```python
from build123d import *

# Parameters (mm, degrees)
SKETCH_1_W             = 162
SKETCH_1_H             = 108
EXTRUDE_1_DEPTH        = 3
SKETCH_2_R             = 2
SKETCH_2_W             = 42
SKETCH_2_H             = 7.5
SKETCH_2_W_2           = 27
SKETCH_2_W_3           = 32
SKETCH_2_W_4           = 58
SKETCH_2_H_2           = 5.8
SKETCH_2_W_5           = 69
SKETCH_2_H_3           = 24
SKETCH_2_W_6           = 13
SKETCH_2_H_4           = 13
CUT_EXTRUDE_2448_DEPTH = 4
FILLET_1_R             = 1.5
SKETCH_3_R             = 1.25
CUT_EXTRUDE_3312_DEPTH = 4
SKETCH_4_R             = 2
CUT_EXTRUDE_4190_DEPTH = 4
FILLET_2_R             = 2


with BuildPart() as part:
    # Эскиз1 → Бобышка-Вытянуть1 (new body)
    with BuildSketch(Plane(origin=(0, 0, 0), x_dir=(1, 0, 0), z_dir=(0, 1, 0))):
        Rectangle(SKETCH_1_W, SKETCH_1_H)
    extrude(amount=EXTRUDE_1_DEPTH)

    # Эскиз2 → Cut-Extrude 2448 (cut, through all)
    with BuildSketch(Plane(origin=(0, 3, 0), x_dir=(1, 0, 0), z_dir=(0, 1, 0))):
        with Locations((-72.99950864, 44.00008818)):
            Circle(SKETCH_2_R)
        with Locations((73, 44)):
            Circle(SKETCH_2_R)
        with Locations((-73, -44)):
            Circle(SKETCH_2_R)
        with Locations((73, -44)):
            Circle(SKETCH_2_R)
        with Locations((-0.725, 38)):
            Rectangle(SKETCH_2_W, SKETCH_2_H)
        with Locations((-31.975, 23)):
            Rectangle(SKETCH_2_W_2, SKETCH_2_H)
        with Locations((31.475, 14)):
            Rectangle(SKETCH_2_W_3, SKETCH_2_H)
        with Locations((0.475, 0)):
            Rectangle(SKETCH_2_W_4, SKETCH_2_H_2)
        with Locations((3, -27)):
            Rectangle(SKETCH_2_W_5, SKETCH_2_H_3)
        with Locations((48.316, -7.9)):
            Rectangle(SKETCH_2_W_6, SKETCH_2_H_4)
    extrude(amount=-CUT_EXTRUDE_2448_DEPTH, mode=Mode.SUBTRACT)

    # Скругление1
    fillet_1_edges = [part.edges().sort_by_distance(p)[0] for p in [
        (-31.5, 1.5, 39),
        (-31.5, 1.5, 15),
        (37.5, 1.5, 15),
        (37.5, 1.5, 39),
    ]]
    fillet(fillet_1_edges, radius=FILLET_1_R)

    # Эскиз3 → Cut-Extrude 3312 (cut, through all)
    with BuildSketch(Plane(origin=(0, 3, 0), x_dir=(1, 0, 0), z_dir=(0, 1, 0))):
        with Locations((-57, 42)):
            Circle(SKETCH_3_R)
        with Locations((-57, -10)):
            Circle(SKETCH_3_R)
        with Locations((60, 42)):
            Circle(SKETCH_3_R)
        with Locations((60, -10)):
            Circle(SKETCH_3_R)
    extrude(amount=-CUT_EXTRUDE_3312_DEPTH, mode=Mode.SUBTRACT)

    # Эскиз4 → Cut-Extrude 4190 (cut, through all)
    with BuildSketch(Plane(origin=(0, 3, 0), x_dir=(1, 0, 0), z_dir=(0, 1, 0))):
        with Locations((-44.5, 2.51)):
            Circle(SKETCH_4_R)
        with Locations((-51.5, 2.51)):
            Circle(SKETCH_4_R)
        with Locations((-49.449747468, 7.459747468)):
            Circle(SKETCH_4_R)
        with Locations((-44.5, 9.51)):
            Circle(SKETCH_4_R)
        with Locations((-39.550252532, 7.459747468)):
            Circle(SKETCH_4_R)
        with Locations((-37.5, 2.51)):
            Circle(SKETCH_4_R)
        with Locations((-39.550252532, -2.439747468)):
            Circle(SKETCH_4_R)
        with Locations((-44.5, -4.49)):
            Circle(SKETCH_4_R)
        with Locations((-49.449747468, -2.439747468)):
            Circle(SKETCH_4_R)
    extrude(amount=-CUT_EXTRUDE_4190_DEPTH, mode=Mode.SUBTRACT)

    # Скругление2
    fillet_2_edges = [part.edges().sort_by_distance(p)[0] for p in [
        (41.816, 1.5, 14.4),
        (41.816, 1.5, 1.4),
        (54.816, 1.5, 1.4),
        (54.816, 1.5, 14.4),
    ]]
    fillet(fillet_2_edges, radius=FILLET_2_R)


solid = part.part
```
Work out the finished part from the listing and answer in its coordinate system (mm). A direction names the side the tool comes from. Round coordinates to 2 decimals unless told otherwise and drop trailing zeros. Loops run counter-clockwise (first coordinate to the right, second up) from the corner with the lowest first, then second, coordinate; pieces in that order, holes last. Notation, with made-up numbers: (77, 27) -> (116, 27) arc R18 ccw to (116, 59) -> close; hole circle Ø3 at (-2.75, -21.75). An arc over 180 degrees is marked (long way). Write each question's results on one line, items separated by ' | '. Start each with the question number.
1. A tool of negligible diameter and unlimited length cuts with its end or side. For faces 1 (the face through (-31.5, 2, 27)), 2 (the face through (-1, 0, -13)), from which of +Z, -Z, +X, -X, +Y, -Y can it reach the whole face along a straight path? Write none if from no direction.
2. Section C-C (z = 44) is taken. Determine the outline of the cut face in (x, y), plus the area to 3 significant figures.
3. Section B-B (z = -25) is taken. Determine the outline of the cut face in (x, y) (3 decimals).
4. Section D-D (x = -7) is taken. Determine the outline of the cut face in (y, z), plus the area to 3 significant figures.
5. Section A-A (x = 33) is taken. Determine the outline of the cut face in (y, z), plus the area to 4 significant figures.
6. For a pull along Z with two mould halves and no side action, classify faces 3 (the face through (-1, 3, -13)), 4 (the face through (-39.498, 1.521, -2.598)), 5 (the face through (-41.55, 1.52, 2.35)), 6 (the face through (-1, 1, 54)) as +Z half, -Z half, draft (parallel to the pull), parting line (faces both ways), or undercut.
7. Find the intervals of material crossed by probe 1 along Z at (x, y) = (-37.5, 1.7); probe 2 along X at (y, z) = (2.4, 44); probe 3 along Z at (x, y) = (-57, 0.8), in increasing order. Write a range as from..to.
Evaluation:
1) face 1: +Y, -Y | face 2: +Z, -Z, +X, -X, -Y
2) outline: (-81, 0) -> (-75, 0) -> (-75, 3) -> (-81, 3) -> close; (-71, 0) -> (71, 0) -> (71, 3) -> (-71, 3) -> close; (75, 0) -> (81, 0) -> (81, 3) -> (75, 3) -> close | area: 462 mm2
3) outline: (-81, 0) -> (-45.475, 0) -> (-45.475, 3) -> (-81, 3) -> close; (-18.475, 0) -> (81, 0) -> (81, 3) -> (-18.475, 3) -> close
4) outline: (0, -54) -> (3, -54) -> (3, -41.75) -> (0, -41.75) -> close; (0, -34.25) -> (3, -34.25) -> (3, -2.9) -> (0, -2.9) -> close; (0, 2.9) -> (3, 2.9) -> (3, 15) -> (0, 15) -> close; (0, 39) -> (3, 39) -> (3, 54) -> (0, 54) -> close | area: 212 mm2
5) outline: (0, -54) -> (3, -54) -> (3, -17.75) -> (0, -17.75) -> close; (0, -10.25) -> (3, -10.25) -> (3, 15) -> (0, 15) -> close; (0, 39) -> (3, 39) -> (3, 54) -> (0, 54) -> close | area: 229.5 mm2
6) face 3: draft | face 4: undercut | face 5: undercut | face 6: +Z half
7) probe 1: z = -54..-26.75, -19.25..-4.51, -0.51..54 | probe 2: x = -81..-75, -71..71, 75..81 | probe 3: z = -54..-43.25, -40.75..8.75, 11.25..54
